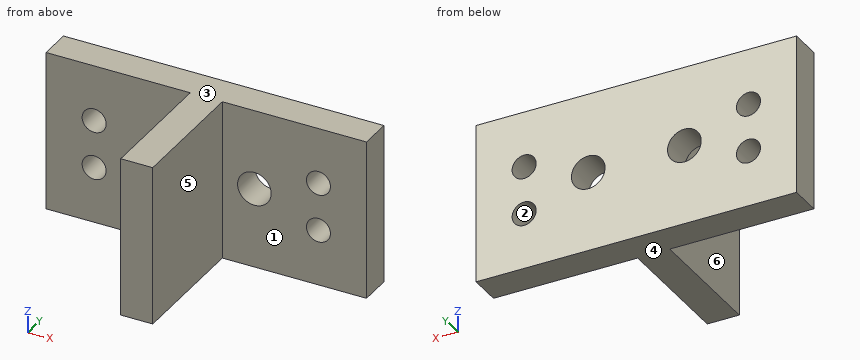
from build123d import *

# Parameters (mm, degrees)
SKETCH_W     = 20
SKETCH_H     = 10
SKETCH_R     = 0.75
SKETCH_R_2   = 1.05
PAD_DEPTH    = 2
SKETCH001_W  = 2
SKETCH001_H  = 10
PAD001_DEPTH = 8


with BuildPart() as part:
    # Sketch → Pad (new body)
    with BuildSketch(Plane.XZ):
        with Locations((10, 5)):
            Rectangle(SKETCH_W, SKETCH_H)
        with Locations((3, 3.5)):
            Circle(SKETCH_R, mode=Mode.SUBTRACT)
        with Locations((3, 6.5)):
            Circle(SKETCH_R, mode=Mode.SUBTRACT)
        with Locations((17, 3.5)):
            Circle(SKETCH_R, mode=Mode.SUBTRACT)
        with Locations((17, 6.5)):
            Circle(SKETCH_R, mode=Mode.SUBTRACT)
        with Locations((7, 5)):
            Circle(SKETCH_R_2, mode=Mode.SUBTRACT)
        with Locations((13, 5)):
            Circle(SKETCH_R_2, mode=Mode.SUBTRACT)
    extrude(amount=PAD_DEPTH)

    # Sketch001 (on Face12 of Pad) → Pad001 (join)
    with BuildSketch(Plane.XZ.offset(2)):
        with Locations((10, 5)):
            Rectangle(SKETCH001_W, SKETCH001_H)
    extrude(amount=PAD001_DEPTH)


solid = part.part
For this review, take the finished solid that the model builds, in its own axes (mm). Face numbers are marked on the shaded views. A direction names the side the tool comes from. Round coordinates to 2 decimals unless told otherwise and drop trailing zeros. Write each loop counter-clockwise with the first axis right and the second up, starting at its lowest first coordinate (ties: lowest second). Pieces come first, ordered by that corner, then holes. Notation, with made-up numbers: (45.25, -40) -> (68.25, -40) arc R10 cw to (68.25, -22) -> close; hole circle Ø5 at (-26.75, 53). An arc over 180 degrees is marked (long way). Put each result on its own line as item: value.
Q1. To check wall thickness, follow L1, parallel to Z at x = 17, y = -0.95; L2, parallel to Z at x = 7, y = -1.1; L3, parallel to Z at x = 3.5, y = -0.5. State the ranges of each line that lie inside material, in increasing order. Write a range as [from, to].
Determined:
L1: z = [0, 2.75], [4.25, 5.75], [7.25, 10]
L2: z = [0, 3.95], [6.05, 10]
L3: z = [0, 2.94], [4.06, 5.94], [7.06, 10]
Q2. Consider section C-C on x = 17. State the section outline as (y, z) points.
Determined:
outline: (-2, 0) -> (0, 0) -> (0, 2.75) -> (-2, 2.75) -> close; (-2, 4.25) -> (0, 4.25) -> (0, 5.75) -> (-2, 5.75) -> close; (-2, 7.25) -> (0, 7.25) -> (0, 10) -> (-2, 10) -> close
Q3. Consider section B-B on x = 13. State the section outline as (y, z) points.
Determined:
outline: (-2, 0) -> (0, 0) -> (0, 3.95) -> (-2, 3.95) -> close; (-2, 6.05) -> (0, 6.05) -> (0, 10) -> (-2, 10) -> close
Q4. Consider section D-D on z = 7.5. State the section outline as (x, y) points, and give its area (3 significant figures).
Determined:
outline: (0, -2) -> (9, -2) -> (9, -10) -> (11, -10) -> (11, -2) -> (20, -2) -> (20, 0) -> (0, 0) -> close
area: 56.0 mm^2
Q5. Clearance check with flat-ended pins moving along their axes: pin 1 Ø1 at (y, z) = (-9, 2) entering from +X; pin 2 Ø6 at (x, y) = (14.5, -3) entering from -Z; pin 3 Ø4 at (y, z) = (-5.5, 3.5) entering from -X; pin 4 Ø4.5 at (x, z) = (13.5, 5.5) entering from -Y. State where each tip first meets the part, or that it passes through.
Determined:
pin 1: stops at x = 11
pin 2: stops at z = 0
pin 3: stops at x = 9
pin 4: stops at y = -2
Q6. Machinability: for the marked faces 4, 5 and 6, which of the approach directions +Z, -Z, +X, -X, +Y, -Y give a long, thin tool a straight path to every point of the face, cutting with its end or side? Answer none if there is none.
Determined:
face 4: -Z, +X, -X, +Y, -Y
face 5: +Z, -Z, +X, -Y
face 6: +Z, -Z, -X, -Y
Q7. Consider section A-A on z = 5. State the section outline as (x, y) points.
Determined:
outline: (0, -2) -> (5.95, -2) -> (5.95, 0) -> (0, 0) -> close; (8.05, -2) -> (9, -2) -> (9, -10) -> (11, -10) -> (11, -2) -> (11.95, -2) -> (11.95, 0) -> (8.05, 0) -> close; (14.05, -2) -> (20, -2) -> (20, 0) -> (14.05, 0) -> close
Q8. The part is to be moulded in two halves that separate along Z. For the marked faces 1, 2 and 3, say which applies: released by +Z, released by -Z, zero draft, split by the parting line, or undercut.
Determined:
face 1: zero draft
face 2: undercut
face 3: released by +Z
